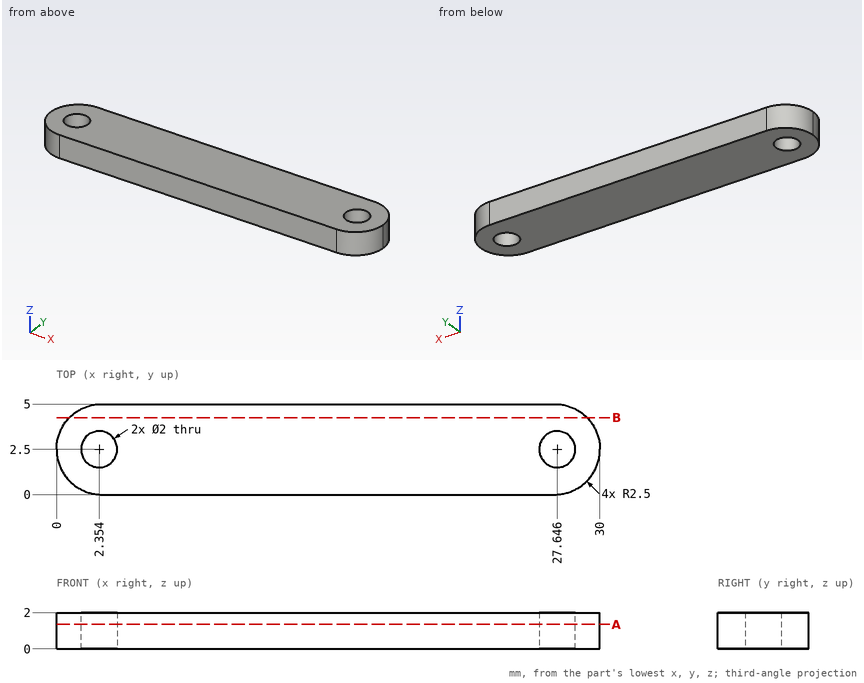
Answer from the drawing. Dimensions are ordinates in mm from the lowest x, y and z of the part. Coordinates: 2 decimals unless noted, no trailing zeros. Loops run counter-clockwise (first coordinate to the right, second up) from the corner with the lowest first, then second, coordinate; pieces in that order, holes last.
Q1. Consider probe 1 along X at (y, z) = (2.6, 0.2); probe 2 along X at (y, z) = (3.35, 0.8); probe 3 along Y at (x, z) = (2, 0.2) (1 decimal). Determine where each line is inside the solid, lowest interval first.
Q2. The part is cut by section A-A on z = 1.35. Give the number of separate pieces and of enclosed holes in the cut face, and give its area (3 significant figures).
Q3. The part is cut by section B-B on y = 4.25. Write down the section's boundary in (x, z).
Results below:
1. probe 1: x = 0 to 1.36, 3.35 to 26.65, 28.64 to 30
1. probe 2: x = 0.15 to 1.83, 2.88 to 27.12, 28.17 to 29.85
1. probe 3: y = 0.1 to 1.6, 3.4 to 4.9
2. separate pieces: 1
2. enclosed holes: 2
2. area: 138 mm2
3. outline: (0.71, 0) - (29.29, 0) - (29.29, 2) - (0.71, 2) - close
